The listing builds one solid part. Answer for the finished solid, in the listing's coordinates (mm). Face numbers are marked on the shaded views. Coordinates: 2 decimals unless noted, no trailing zeros. Loops run counter-clockwise (first coordinate to the right, second up) from the corner with the lowest first, then second, coordinate; pieces in that order, holes last. Notation, with made-up numbers: (82.25, 12.5) - (113.25, 12.5) arc R29 ccw to (113.25, 35.5) - close; hole circle Ø4 at (57, -13). An arc over 180 degrees is marked (long way). Put each result on its own line as item: value.
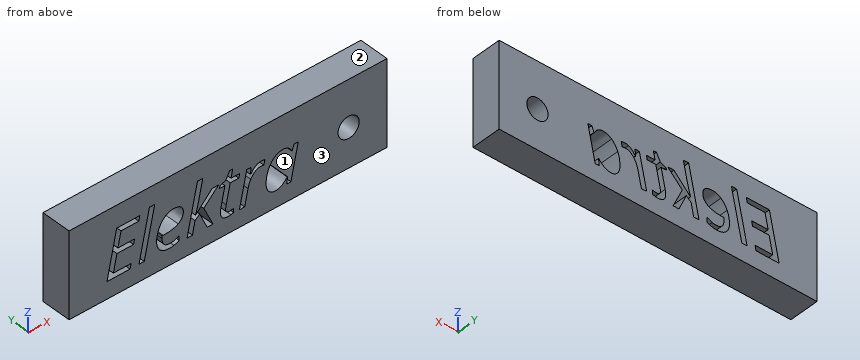
```python
from build123d import *

# Parameters (mm, degrees)
F0_W     = 75
F0_H     = 20
F0_R     = 2.5
F1_DEPTH = 7


with BuildPart() as f1:
    # F0 (on Front) → F1 (new body)
    with BuildSketch(Plane.XZ):
        with Locations((37.5, -10)):
            Rectangle(F0_W, F0_H)
        Polygon((14.6358500468, -14.8998533473), (14.3914699527, -16.0268489271), (8.941556591, -16.0268489271), (11.2311370847, -5.1863377606), (16.6810504464, -5.1863377606), (16.4437882191, -6.3204512072), (12.2489920399, -6.3204512072), (11.520597002, -9.7987154598), (15.4283058861, -9.7987154598), (15.2147698815, -10.9257110396), (11.2904526415, -10.9257110396), (10.4457991123, -14.8998533473), align=None, mode=Mode.SUBTRACT)
        Polygon((20.1972766554, -4.4887868122), (17.7344947357, -16.0268489271), (16.4888680423, -16.0268489271), (18.9516499619, -4.4887868122), align=None, mode=Mode.SUBTRACT)
        with BuildLine():
            add(Edge.make_bspline(
                [(24.7479661755, -16.0458299053), (24.214126164, -16.1763241304), (23.571145528, -16.1763241304)],
                knots=[0, 0, 0, 1, 1, 1], degree=2))
            add(Edge.make_bspline(
                [(23.571145528, -16.1763241304), (22.2068877208, -16.1763241304), (21.4274813041, -15.3672599352)],
                knots=[0, 0, 0, 1, 1, 1], degree=2))
            add(Edge.make_bspline(
                [(21.4274813041, -15.3672599352), (20.6480748873, -14.55819574), (20.6480748873, -13.1275045092)],
                knots=[0, 0, 0, 1, 1, 1], degree=2))
            add(Edge.make_bspline(
                [(20.6480748873, -13.1275045092), (20.6480748873, -11.7347752348), (21.200895877, -10.4547455184)],
                knots=[0, 0, 0, 1, 1, 1], degree=2))
            add(Edge.make_bspline(
                [(21.200895877, -10.4547455184), (21.7537168666, -9.1747158019), (22.6659901307, -8.46292912)],
                knots=[0, 0, 0, 1, 1, 1], degree=2))
            add(Edge.make_bspline(
                [(22.6659901307, -8.46292912), (23.5782633948, -7.751142438), (24.674414885, -7.751142438)],
                knots=[0, 0, 0, 1, 1, 1], degree=2))
            add(Edge.make_bspline(
                [(24.674414885, -7.751142438), (25.8085283317, -7.751142438), (26.3803302995, -8.2446478708)],
                knots=[0, 0, 0, 1, 1, 1], degree=2))
            add(Edge.make_bspline(
                [(26.3803302995, -8.2446478708), (26.9521322674, -8.7381533037), (26.9521322674, -9.6207687893)],
                knots=[0, 0, 0, 1, 1, 1], degree=2))
            add(Edge.make_bspline(
                [(26.9521322674, -9.6207687893), (26.9521322674, -10.9541825069), (25.7207413075, -11.7146079455)],
                knots=[0, 0, 0, 1, 1, 1], degree=2))
            add(Edge.make_bspline(
                [(25.7207413075, -11.7146079455), (24.4893503477, -12.4750333841), (22.1973972317, -12.4750333841)],
                knots=[0, 0, 0, 1, 1, 1], degree=2))
            Line((22.1973972317, -12.4750333841), (21.9530171376, -12.4750333841))
            Line((21.9530171376, -12.4750333841), (21.9245456703, -13.0681889524))
            add(Edge.make_bspline(
                [(21.9245456703, -13.0681889524), (21.9245456703, -14.0385914621), (22.3800891468, -14.584294585)],
                knots=[0, 0, 0, 1, 1, 1], degree=2))
            add(Edge.make_bspline(
                [(22.3800891468, -14.584294585), (22.8356326233, -15.1299977078), (23.7917993994, -15.1299977078)],
                knots=[0, 0, 0, 1, 1, 1], degree=2))
            add(Edge.make_bspline(
                [(23.7917993994, -15.1299977078), (24.2592059872, -15.1299977078), (24.7527114201, -14.9959445494)],
                knots=[0, 0, 0, 1, 1, 1], degree=2))
            add(Edge.make_bspline(
                [(24.7527114201, -14.9959445494), (25.2462168529, -14.861891391), (25.9793571353, -14.50599805)],
                knots=[0, 0, 0, 1, 1, 1], degree=2))
            Line((25.9793571353, -14.50599805), (25.9793571353, -15.5902864289))
            add(Edge.make_bspline(
                [(25.9793571353, -15.5902864289), (25.281806187, -15.9153356803), (24.7479661755, -16.0458299053)],
                knots=[0, 0, 0, 1, 1, 1], degree=2))
        make_face(mode=Mode.SUBTRACT)
        with BuildLine():
            Line((29.8277504626, -11.8818778157), (29.8562219299, -11.8818778157))
            Line((29.8562219299, -11.8818778157), (33.7568129471, -7.9006176412))
            Line((33.7568129471, -7.9006176412), (35.2468197347, -7.9006176412))
            Line((35.2468197347, -7.9006176412), (31.7709281044, -11.3622735379))
            Line((31.7709281044, -11.3622735379), (33.9561132181, -16.0268489271))
            Line((33.9561132181, -16.0268489271), (32.5705018105, -16.0268489271))
            Line((32.5705018105, -16.0268489271), (30.8289970619, -12.1404936435))
            Line((30.8289970619, -12.1404936435), (29.7020014821, -13.0539532187))
            Line((29.7020014821, -13.0539532187), (29.0922375579, -16.0268489271))
            Line((29.0922375579, -16.0268489271), (27.8323751308, -16.0268489271))
            Line((27.8323751308, -16.0268489271), (30.2785486945, -4.4887868122))
            Line((30.2785486945, -4.4887868122), (31.5407837439, -4.4887868122))
            add(Edge.make_bspline(
                [(31.5407837439, -4.4887868122), (31.0069437324, -6.9800401992), (30.5834306566, -8.9528756194)],
                knots=[0, 0, 0, 1, 1, 1], degree=2))
            add(Edge.make_bspline(
                [(30.5834306566, -8.9528756194), (30.1599175808, -10.9257110396), (29.8277504626, -11.8818778157)],
                knots=[0, 0, 0, 1, 1, 1], degree=2))
        make_face(mode=Mode.SUBTRACT)
        with BuildLine():
            add(Edge.make_bspline(
                [(44.4668298886, -7.9184123082), (44.8488220746, -7.751142438), (45.3162286625, -7.751142438)],
                knots=[0, 0, 0, 1, 1, 1], degree=2))
            add(Edge.make_bspline(
                [(45.3162286625, -7.751142438), (45.8287150735, -7.751142438), (46.2059620149, -7.855537818)],
                knots=[0, 0, 0, 1, 1, 1], degree=2))
            Line((46.2059620149, -7.855537818), (45.9402283203, -8.9682976642))
            add(Edge.make_bspline(
                [(45.9402283203, -8.9682976642), (45.546373023, -8.871020151), (45.1596355924, -8.871020151)],
                knots=[0, 0, 0, 1, 1, 1], degree=2))
            add(Edge.make_bspline(
                [(45.1596355924, -8.871020151), (44.4858108668, -8.871020151), (43.8962142319, -9.3158868272)],
                knots=[0, 0, 0, 1, 1, 1], degree=2))
            add(Edge.make_bspline(
                [(43.8962142319, -9.3158868272), (43.306617597, -9.7607535034), (42.8653098542, -10.5508367204)],
                knots=[0, 0, 0, 1, 1, 1], degree=2))
            add(Edge.make_bspline(
                [(42.8653098542, -10.5508367204), (42.4240021113, -11.3409199374), (42.2175839736, -12.3042045804)],
                knots=[0, 0, 0, 1, 1, 1], degree=2))
            Line((42.2175839736, -12.3042045804), (41.422755512, -16.0268489271))
            Line((41.422755512, -16.0268489271), (40.1771288186, -16.0268489271))
            Line((40.1771288186, -16.0268489271), (41.9138883226, -7.9006176412))
            Line((41.9138883226, -7.9006176412), (42.9436063892, -7.9006176412))
            Line((42.9436063892, -7.9006176412), (42.7798954523, -9.4048601625))
            Line((42.7798954523, -9.4048601625), (42.8558193651, -9.4048601625))
            add(Edge.make_bspline(
                [(42.8558193651, -9.4048601625), (43.3896593766, -8.7001913473), (43.7372485396, -8.3929367629)],
                knots=[0, 0, 0, 1, 1, 1], degree=2))
            add(Edge.make_bspline(
                [(43.7372485396, -8.3929367629), (44.0848377026, -8.0856821785), (44.4668298886, -7.9184123082)],
                knots=[0, 0, 0, 1, 1, 1], degree=2))
        make_face(mode=Mode.SUBTRACT)
        with BuildLine():
            add(Edge.make_bspline(
                [(37.1461038645, -14.9366289926), (37.3608261802, -15.1584691751), (37.7451909885, -15.1584691751)],
                knots=[0, 0, 0, 1, 1, 1], degree=2))
            add(Edge.make_bspline(
                [(37.7451909885, -15.1584691751), (38.1532820195, -15.1584691751), (38.8128710114, -14.966286771)],
                knots=[0, 0, 0, 1, 1, 1], degree=2))
            Line((38.8128710114, -14.966286771), (38.8128710114, -15.9224535471))
            add(Edge.make_bspline(
                [(38.8128710114, -15.9224535471), (38.5613730505, -16.0268489271), (38.1912439758, -16.1015865287)],
                knots=[0, 0, 0, 1, 1, 1], degree=2))
            add(Edge.make_bspline(
                [(38.1912439758, -16.1015865287), (37.8211149012, -16.1763241304), (37.5980884075, -16.1763241304)],
                knots=[0, 0, 0, 1, 1, 1], degree=2))
            add(Edge.make_bspline(
                [(37.5980884075, -16.1763241304), (36.6703930987, -16.1763241304), (36.178073977, -15.7350163875)],
                knots=[0, 0, 0, 1, 1, 1], degree=2))
            add(Edge.make_bspline(
                [(36.178073977, -15.7350163875), (35.6857548553, -15.2937086447), (35.6857548553, -14.4182110259)],
                knots=[0, 0, 0, 1, 1, 1], degree=2))
            add(Edge.make_bspline(
                [(35.6857548553, -14.4182110259), (35.6857548553, -13.9294508376), (35.8186217026, -13.3054511797)],
                knots=[0, 0, 0, 1, 1, 1], degree=2))
            Line((35.8186217026, -13.3054511797), (36.7605527451, -8.8425486837))
            Line((36.7605527451, -8.8425486837), (35.484081962, -8.8425486837))
            Line((35.484081962, -8.8425486837), (35.5884773421, -8.3015908054))
            Line((35.5884773421, -8.3015908054), (36.959853016, -7.7226709707))
            Line((36.959853016, -7.7226709707), (37.8875483249, -6.0309912899))
            Line((37.8875483249, -6.0309912899), (38.6135707405, -6.0309912899))
            Line((38.6135707405, -6.0309912899), (38.2054797095, -7.9006176412))
            Line((38.2054797095, -7.9006176412), (40.2364443754, -7.9006176412))
            Line((40.2364443754, -7.9006176412), (40.0442619713, -8.8425486837))
            Line((40.0442619713, -8.8425486837), (38.0204151722, -8.8425486837))
            Line((38.0204151722, -8.8425486837), (37.064248396, -13.3196869133))
            add(Edge.make_bspline(
                [(37.064248396, -13.3196869133), (36.9313815487, -13.9650401717), (36.9313815487, -14.2995799122)],
                knots=[0, 0, 0, 1, 1, 1], degree=2))
            add(Edge.make_bspline(
                [(36.9313815487, -14.2995799122), (36.9313815487, -14.71478881), (37.1461038645, -14.9366289926)],
                knots=[0, 0, 0, 1, 1, 1], degree=2))
        make_face(mode=Mode.SUBTRACT)
        with BuildLine():
            add(Edge.make_bspline(
                [(48.4587668634, -8.5008910763), (49.3852758611, -7.751142438), (50.4909178405, -7.751142438)],
                knots=[0, 0, 0, 1, 1, 1], degree=2))
            add(Edge.make_bspline(
                [(50.4909178405, -7.751142438), (51.1718604329, -7.751142438), (51.7057004444, -8.1188988903)],
                knots=[0, 0, 0, 1, 1, 1], degree=2))
            add(Edge.make_bspline(
                [(51.7057004444, -8.1188988903), (52.2395404559, -8.4866553427), (52.53611824, -9.1747158019)],
                knots=[0, 0, 0, 1, 1, 1], degree=2))
            Line((52.53611824, -9.1747158019), (52.6191600196, -9.1747158019))
            Line((52.6191600196, -9.1747158019), (53.1150380747, -7.9006176412))
            Line((53.1150380747, -7.9006176412), (54.0569691172, -7.9006176412))
            Line((54.0569691172, -7.9006176412), (52.3297001022, -16.0268489271))
            Line((52.3297001022, -16.0268489271), (51.3426892366, -16.0268489271))
            Line((51.3426892366, -16.0268489271), (51.537244263, -14.4775265827))
            Line((51.537244263, -14.4775265827), (51.4779287061, -14.4775265827))
            add(Edge.make_bspline(
                [(51.4779287061, -14.4775265827), (50.1492602331, -16.1763241304), (48.680607046, -16.1763241304)],
                knots=[0, 0, 0, 1, 1, 1], degree=2))
            add(Edge.make_bspline(
                [(48.680607046, -16.1763241304), (47.6508889794, -16.1763241304), (47.0648512779, -15.4419975368)],
                knots=[0, 0, 0, 1, 1, 1], degree=2))
            add(Edge.make_bspline(
                [(47.0648512779, -15.4419975368), (46.4788135764, -14.7076709432), (46.4788135764, -13.4312001602)],
                knots=[0, 0, 0, 1, 1, 1], degree=2))
            add(Edge.make_bspline(
                [(46.4788135764, -13.4312001602), (46.4788135764, -11.8889956826), (47.005535721, -10.5698176986)],
                knots=[0, 0, 0, 1, 1, 1], degree=2))
            add(Edge.make_bspline(
                [(47.005535721, -10.5698176986), (47.5322578657, -9.2506397147), (48.4587668634, -8.5008910763)],
                knots=[0, 0, 0, 1, 1, 1], degree=2))
        make_face(mode=Mode.SUBTRACT)
        with Locations((65.950281918, -10.8088040724)):
            Circle(F0_R, mode=Mode.SUBTRACT)
    extrude(amount=F1_DEPTH)


solid = f1.part
```
1) For a pull along Z with two mould halves and no side action, classify the marked faces 1, 2 and 3 as pulls with the +Z half, pulls with the -Z half, needs draft (parallel to the pull), parting line crosses it, or undercut.
Found:
face 1: undercut
face 2: pulls with the +Z half
face 3: needs draft
2) The part is cut by section B-B (y = -1.75). State how many separate pieces and enclosed holes the cut face has, and give its area (3 significant figures).
Found:
separate pieces: 1
enclosed holes: 8
area: 1,300 mm^2
3) This flat-tipped pin is pushed along its axis until it touches: pin 1 (4.5 mm diameter, centred on x = 65.95, z = -10.81, fed in from -Y). Where does it stop, or does it pass through?
Found:
pin 1: passes through
4) Straight lines are drawn through the part: L1, parallel to Z at x = 13, y = -3.5; L2, parallel to X at y = -1.25, z = -6.5; L3, parallel to X at y = -1.75, z = -4.75. For each, find the intervals that lie inside material, in ascending order. Write a range as [from, to].
Found:
L1: z = [-20, -16.03], [-14.9, -10.93], [-9.8, -6.32], [-5.19, 0]
L2: x = [0, 10.95], [12.21, 18.52], [19.77, 29.85], [31.11, 37.63], [38.51, 75]
L3: x = [0, 18.9], [20.14, 30.22], [31.48, 75]
5) The part is cut by section A-A (x = 67). Give the vertices of the cut face in (y, z), and give its area (3 significant figures).
Found:
outline: (-7, -20) - (0, -20) - (0, -13.08) - (-7, -13.08) - close; (-7, -8.54) - (0, -8.54) - (0, 0) - (-7, 0) - close
area: 108 mm^2
